```python
from build123d import *

# Parameters (mm, degrees)
F0_R     = 3
F0_R_2   = 2.5
F1_DEPTH = 1000
F2_R     = 2
F3_R     = 7
F5_DEPTH = 30


# Not quite as in the source:
# - a feature names something its author has since deleted; it is built from what else it names


with BuildPart() as f1:
    # F0 (on Top) → F1 (new body)
    with BuildSketch(Plane.XY):
        with BuildLine():
            Line((18.15, -15), (30, -15))
            Line((30, -15), (30, -3.15))
            Line((30, -3.15), (27.5, -3.15))
            Line((27.5, -3.15), (27.5, -5.15))
            Line((27.5, -5.15), (21.5477069044, -5.15))
            ThreePointArc((21.5477069044, -5.15), (19.5, 0), (21.5477069044, 5.15))
            Line((21.5477069044, 5.15), (27.5, 5.15))
            Line((27.5, 5.15), (27.5, 3.15))
            Line((27.5, 3.15), (30, 3.15))
            Line((30, 3.15), (30, 15))
            Line((30, 15), (18.15, 15))
            Line((18.15, 15), (18.15, 12.5))
            Line((18.15, 12.5), (20.15, 12.5))
            Line((20.15, 12.5), (20.15, 6.5477069044))
            ThreePointArc((20.15, 6.5477069044), (15, 4.5), (9.85, 6.5477069044))
            Line((9.85, 6.5477069044), (9.85, 12.5))
            Line((9.85, 12.5), (11.85, 12.5))
            Line((11.85, 12.5), (11.85, 15))
            Line((11.85, 15), (-11.85, 15))
            Line((-11.85, 15), (-11.85, 12.5))
            Line((-11.85, 12.5), (-9.85, 12.5))
            Line((-9.85, 12.5), (-9.85, 6.5477069044))
            ThreePointArc((-9.85, 6.5477069044), (-15, 4.5), (-20.15, 6.5477069044))
            Line((-20.15, 6.5477069044), (-20.15, 12.5))
            Line((-20.15, 12.5), (-18.15, 12.5))
            Line((-18.15, 12.5), (-18.15, 15))
            Line((-18.15, 15), (-30, 15))
            Line((-30, 15), (-30, 3.15))
            Line((-30, 3.15), (-27.5, 3.15))
            Line((-27.5, 3.15), (-27.5, 5.15))
            Line((-27.5, 5.15), (-21.5477069044, 5.15))
            ThreePointArc((-21.5477069044, 5.15), (-19.5, 0), (-21.5477069044, -5.15))
            Line((-21.5477069044, -5.15), (-27.5, -5.15))
            Line((-27.5, -5.15), (-27.5, -3.15))
            Line((-27.5, -3.15), (-30, -3.15))
            Line((-30, -3.15), (-30, -15))
            Line((-30, -15), (-18.15, -15))
            Line((-18.15, -15), (-18.15, -12.5))
            Line((-18.15, -12.5), (-20.15, -12.5))
            Line((-20.15, -12.5), (-20.15, -6.5477069044))
            ThreePointArc((-20.15, -6.5477069044), (-15, -4.5), (-9.85, -6.5477069044))
            Line((-9.85, -6.5477069044), (-9.85, -12.5))
            Line((-9.85, -12.5), (-11.85, -12.5))
            Line((-11.85, -12.5), (-11.85, -15))
            Line((-11.85, -15), (11.85, -15))
            Line((11.85, -15), (11.85, -12.5))
            Line((11.85, -12.5), (9.85, -12.5))
            Line((9.85, -12.5), (9.85, -6.5477069044))
            ThreePointArc((9.85, -6.5477069044), (15, -4.5), (20.15, -6.5477069044))
            Line((20.15, -6.5477069044), (20.15, -12.5))
            Line((20.15, -12.5), (18.15, -12.5))
            Line((18.15, -12.5), (18.15, -15))
        make_face()
        with Locations((-25, -10)):
            Circle(F0_R, mode=Mode.SUBTRACT)
        with Locations((25, -10)):
            Circle(F0_R, mode=Mode.SUBTRACT)
        with Locations((-15, 0)):
            Circle(F0_R_2, mode=Mode.SUBTRACT)
        with Locations((-25, 10)):
            Circle(F0_R, mode=Mode.SUBTRACT)
        Polygon((-7, 7), (-7, 12.5), (0, 12.5), (7, 12.5), (7, 7), (10, 0), (7, -7), (7, -12.5), (0, -12.5), (-7, -12.5), (-7, -7), (-10, 0), align=None, mode=Mode.SUBTRACT)
        with Locations((15, 0)):
            Circle(F0_R_2, mode=Mode.SUBTRACT)
        with Locations((25, 10)):
            Circle(F0_R, mode=Mode.SUBTRACT)
    extrude(amount=F1_DEPTH)

    # F2
    f2_edges = [f1.edges().sort_by_distance(p)[0] for p in [
        (-7, 12.5, 500),
        (7, 12.5, 500),
    ]]
    fillet(f2_edges, radius=F2_R)

    # F3
    f3_edges = [f1.edges().sort_by_distance(p)[0] for p in [
        (-7, 7, 500),
        (-10, 0, 500),
        (7, 7, 500),
        (10, 0, 500),
    ]]
    fillet(f3_edges, radius=F3_R)

    # F4 (on Right) → F5 (cut, symmetric)
    with BuildSketch(Plane.YZ):
        Polygon((15, 30), (-15, 0), (15, 0), align=None)
        Polygon((15, 1000), (-15, 1000), (15, 970), align=None)
    extrude(amount=F5_DEPTH, both=True, mode=Mode.SUBTRACT)


solid = f1.part
```
Design review of the part built by this model. Coordinates are the model's own, in mm. Coordinates: 2 decimals unless noted, no trailing zeros.
1) To check wall thickness, follow L1, parallel to Y at x = 25, z = 273.5; L2, parallel to X at y = 0, z = 337.5; L3, parallel to X at y = 13.5, z = 937.5. State the ranges of each line that lie inside material, in increasing order.
2) Add section A-A (z = 277.5). State how many separate pieces and enclosed holes the cut face has, plus the area to 3 significant figures.
3) Insertion check: pin 1 (6.5 mm diameter, centred on x = 15, y = 0, fed in from -Z); pin 2 (2 mm diameter, centred on x = -24, y = -4.5, fed in from +Z); pin 3 (6 mm diameter, centred on x = -10.5, y = -3.5, fed in from +Z). Each pin has a flat end and moves straight along its axis. Give the tip position at first contact, or say it passes through.
Check result:
1. L1: y = -15 to -13, -7 to -5.15, 5.15 to 7, 13 to 15
1. L2: x = -19.5 to -17.5, -12.5 to -9.38, 9.38 to 12.5, 17.5 to 19.5
1. L3: x = -30 to -18.15, -11.85 to 11.85, 18.15 to 30
2. separate pieces: 1
2. enclosed holes: 7
2. area: 710 mm2
3. pin 1: stops at z = 11.75
3. pin 2: stops at z = 990.5
3. pin 3: stops at z = 991.45
